```python
from build123d import *

# Parameters (mm, degrees)
F0_W     = 20
F0_H     = 20
F1_DEPTH = 8
F3_DEPTH = 4
F5_DEPTH = 19
F6_W     = 6
F6_H     = 8
F7_DEPTH = 7
F8_R     = 2.2
F9_DEPTH = 6


with BuildPart() as f1:
    # F0 (on Top) → F1 (new body)
    with BuildSketch(Plane.XY):
        Rectangle(F0_W, F0_H)
    extrude(amount=F1_DEPTH)

    # F2 (on face) → F3 (cut)
    with BuildSketch(Plane(origin=(0, 0, 0), x_dir=(1, 0, 0), z_dir=(0, 0, -1))):
        with BuildLine():
            ThreePointArc((6.430839, -0.945677), (6.482687, -0.474101), (6.5, 0))
            ThreePointArc((6.5, 0), (-0.474101, 6.482687), (-6.430839, -0.945677))
            Line((-6.430839, -0.945677), (6.430839, -0.945677))
        make_face()
        with BuildLine():
            Line((6.430839, -0.945677), (-6.430839, -0.945677))
            ThreePointArc((-6.430839, -0.945677), (0, -6.5), (6.430839, -0.945677))
        make_face()
        with BuildLine():
            ThreePointArc((6.430839, -0.945677), (0, -6.5), (-6.430839, -0.945677))
            Line((-6.430839, -0.945677), (-6.430839, -10))
            Line((-6.430839, -10), (6.430839, -10))
            Line((6.430839, -10), (6.430839, -0.945677))
        make_face()
    extrude(amount=-F3_DEPTH, mode=Mode.SUBTRACT)

    # F4 (on face) → F5 (cut)
    with BuildSketch(Plane(origin=(0, 10, 0), x_dir=(-1, 0, 0), z_dir=(0, 1, 0))):
        Polygon((6.430839, 4), (9.473302, 4), (9.473302, 6.210144), (-9.087299, 6.210144), (-9.087299, 4), (-6.430839, 4), align=None)
    extrude(amount=-F5_DEPTH, mode=Mode.SUBTRACT)

    # F6 (on face) → F7 (join)
    with BuildSketch(Plane.XY.offset(8)):
        Rectangle(F6_W, F6_H)
    extrude(amount=F7_DEPTH)

    # F8 (on face) → F9 (cut)
    with BuildSketch(Plane(origin=(-3, 0, 0), x_dir=(0, -1, 0), z_dir=(-1, 0, 0))):
        with Locations((0, 11)):
            Circle(F8_R)
    extrude(amount=-F9_DEPTH, mode=Mode.SUBTRACT)


solid = f1.part
```
Build history of the part. All positions in model axes, mm. A direction names the side the tool comes from. Coordinates: 2 decimals unless noted, no trailing zeros. Order: outer loops, then holes, each group sorted by start corner. A loop starts at its lowest first (then second) coordinate and runs counter-clockwise, first axis right, second up. Notation, with made-up numbers: M 25.5,-31 L 53.5,-31 A16 ccw 53.5,-3 Z; hole C 8,83.25 d6. An arc over 180 degrees is marked long. One line per question, with ' | ' between items. Start each with the question number.
1. Cut at B-B (y = -8.25). Write the cut outline in (x, z), plus the area to 3 significant figures.
2. Cut at C-C (x = 7). Write the cut outline in (y, z).
3. Wall check: line 1 along X through (y, z) = (7.75, 2.5); line 2 along Z through (x, y) = (0.75, 0); line 3 along Z through (x, y) = (-7.25, -5.5). Give the ranges that are in metal, low to high. Write a range as [from, to].
4. Cut at A-A (z = 11). Write the cut outline in (x, y), plus the area to 3 significant figures.
5. Cut at D-D (z = 5.5). Write the cut outline in (x, y).
6. Tool access for faces 1 (the face through (6.431, 6, 2)), 2 (the face through (0, 4, 11)), 3 (the face through (9.087, 1, 5)): list every direction of +Z, -Z, +X, -X, +Y, -Y with a clear straight run to the whole face (end or side of a thin tool).
7. Mould opens along Y. For faces 4 (the face through (-10, 0, 4)), 5 (the face through (0, -4, 11)), 6 (the face through (0, 10, 7)), 7 (the face through (-0.042, -1.183, 12.855)) say: +Y half, -Y half, draft (parallel to the pull), parting line (faces both ways), or undercut.
8. Flat gauge pins, fed straight in: P1, Ø3, axis at x = 2, y = 6, coming from the -Z side; P2, Ø7.5, axis at y = 0, z = 12, coming from the +X side; P3, Ø5, axis at x = 0.5, z = 13, coming from the +Y side. Where does each tip first touch, or does it go through?
The answers:
1) outline: M -10,0 L 10,0 L 10,8 L -10,8 Z; hole M -9.47,4 L 9.09,4 L 9.09,6.21 L -9.47,6.21 Z | area: 119 mm2
2) outline: M -10,0 L 10,0 L 10,4 L -9,4 L -9,6.21 L 10,6.21 L 10,8 L -10,8 Z
3) line 1: x = [-10, -6.43], [6.43, 10] | line 2: z = [6.21, 8.8], [13.2, 15] | line 3: z = [0, 4], [6.21, 8]
4) outline: M -3,-4 L 3,-4 L 3,-2.2 L -3,-2.2 Z; M -3,2.2 L 3,2.2 L 3,4 L -3,4 Z | area: 21.6 mm2
5) outline: M -10,-10 L 10,-10 L 10,10 L 9.09,10 L 9.09,-9 L -9.47,-9 L -9.47,10 L -10,10 Z
6) face 1: -Z, +Y | face 2: +Z, +X, -X, +Y | face 3: +Y
7) face 4: draft | face 5: -Y half | face 6: +Y half | face 7: undercut
8) P1: stops at z = 6.21 | P2: stops at x = 3 | P3: stops at y = 4
